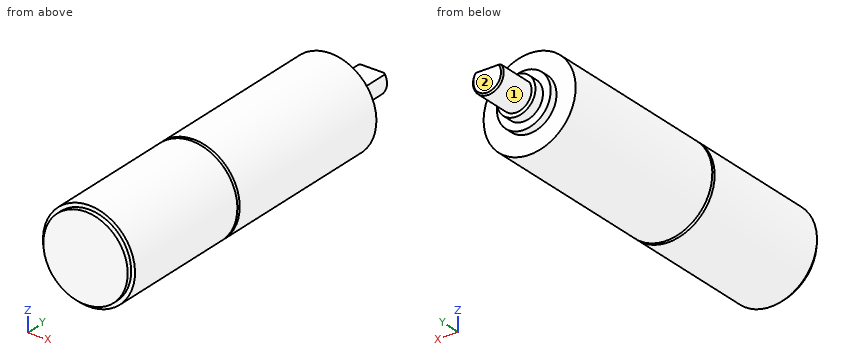
from build123d import *

# Parameters (mm, degrees)
SKETCH_1_R          = 2.75
EXTRUDE_1_DEPTH     = 0.3
EXTRUDE_START       = 0.3
SKETCH_2_R          = 3
EXTRUDE_2_DEPTH     = 9
CHAMFER_1_SIZE      = 0.2
EXTRUDE_START_2     = 9.3
SKETCH_3_R          = 3
EXTRUDE_3_DEPTH     = 11.75
EXTRUDE_START_3     = 21.05
SKETCH_4_R          = 1.75
EXTRUDE_4_DEPTH     = 0.5
SKETCH_5_R          = 1.25
EXTRUDE_5_DEPTH     = 1.15
SKETCH_6_R          = 1
EXTRUDE_6_DEPTH     = 3.65
CUT_EXTRUDE_START   = 22.2
CUT_EXTRUDE_1_DEPTH = 2.5
CHAMFER_2_SIZE      = 0.1


with BuildPart() as part:
    # 草图1 → 凸台-拉伸1 (new body)
    with BuildSketch(Plane(origin=(0, 0, 0), x_dir=(1, 0, 0), z_dir=(0, 1, 0))):
        with Locations(Location((0, 0, 0), (0, 0, 270))):
            Circle(SKETCH_1_R)
    extrude(amount=EXTRUDE_1_DEPTH)

    # 草图2 → 凸台-拉伸2 (add)
    with BuildSketch(Plane(origin=(0, 0, 0), x_dir=(1, 0, 0), z_dir=(0, 1, 0)).offset(EXTRUDE_START)):
        with Locations(Location((0, 0, 0), (0, 0, 270))):
            Circle(SKETCH_2_R)
    extrude(amount=EXTRUDE_2_DEPTH)

    # 倒角1
    chamfer_1_edges = [part.edges().sort_by_distance(p)[0] for p in [
        (0, 9.3, -3),
    ]]
    chamfer(chamfer_1_edges, length=CHAMFER_1_SIZE)

    # 草图3 → 凸台-拉伸3 (add)
    with BuildSketch(Plane(origin=(0, 0, 0), x_dir=(1, 0, 0), z_dir=(0, 1, 0)).offset(EXTRUDE_START_2)):
        with Locations(Location((0, 0, 0), (0, 0, 270))):
            Circle(SKETCH_3_R)
    extrude(amount=EXTRUDE_3_DEPTH)

    # 草图4 → 凸台-拉伸4 (add)
    with BuildSketch(Plane(origin=(0, 0, 0), x_dir=(1, 0, 0), z_dir=(0, 1, 0)).offset(EXTRUDE_START_3)):
        with Locations(Location((0, 0, 0), (0, 0, 270))):
            Circle(SKETCH_4_R)
    extrude(amount=EXTRUDE_4_DEPTH)

    # 草图5 → 凸台-拉伸5 (add)
    with BuildSketch(Plane(origin=(0, 0, 0), x_dir=(1, 0, 0), z_dir=(0, 1, 0)).offset(EXTRUDE_START_3)):
        with Locations(Location((0, 0, 0), (0, 0, 270))):
            Circle(SKETCH_5_R)
    extrude(amount=EXTRUDE_5_DEPTH)

    # 草图6 → 凸台-拉伸6 (add)
    with BuildSketch(Plane(origin=(0, 0, 0), x_dir=(1, 0, 0), z_dir=(0, 1, 0)).offset(EXTRUDE_START_3)):
        with Locations(Location((0, 0, 0), (0, 0, 270))):
            Circle(SKETCH_6_R)
    extrude(amount=EXTRUDE_6_DEPTH)

    # 草图7 → 切除-拉伸1 (cut)
    with BuildSketch(Plane(origin=(0, 0, 0), x_dir=(1, 0, 0), z_dir=(0, 1, 0)).offset(CUT_EXTRUDE_START)):
        with BuildLine():
            Line((-0.866025404, -0.5), (0.866025404, -0.5))
            ThreePointArc((0.866025404, -0.5), (0, -1), (-0.866025404, -0.5))
        make_face()
    extrude(amount=CUT_EXTRUDE_1_DEPTH, mode=Mode.SUBTRACT)

    # 倒角2
    chamfer_2_edges = [part.edges().sort_by_distance(p)[0] for p in [
        (0, 24.7, -1),
    ]]
    chamfer(chamfer_2_edges, length=CHAMFER_2_SIZE)


solid = part.part
CAD build for the part. Positions are in the model's coordinates, mm. Face numbers are marked on the shaded views. A direction names the side the tool comes from. Coordinates: 2 decimals unless noted, no trailing zeros. Order: outer loops, then holes, each group sorted by start corner. A loop starts at its lowest first (then second) coordinate and runs counter-clockwise, first axis right, second up. Notation, with made-up numbers: (-39.5, 38.25) -> (-22.5, 38.25) arc R11 ccw to (-22.5, 42.25) -> close; hole circle Ø2 at (55, 50). An arc over 180 degrees is marked (long way). Answer in a Markdown table with one row per item.
1) Band-saw the part on C-C (y = 7). List the corners of the cut face in (x, z).
Check values:
| item | result |
|---|---|
| outline | circle Ø6 at (0, 0) |
2) Flat gauge pins, fed straight in: P1, Ø2, axis at y = 16, z = 2, coming from the -X side; P2, Ø1.5, axis at y = 11.5, z = 1.5, coming from the +X side; P3, Ø1, axis at x = -1.5, y = 6.5, coming from the -Z side. Where does each tip first touch, or does it go through?
Check values:
| item | result |
|---|---|
| P1 | x = -2.83 |
| P2 | x = 2.9 |
| P3 | z = -2.83 |
3) Band-saw the part on A-A (z = 0). List the corners of the cut face in (x, y), and give its area (3 significant figures).
Check values:
| item | result |
|---|---|
| outline | (-3, 0.3) -> (-2.75, 0.3) -> (-2.75, 0) -> (2.75, 0) -> (2.75, 0.3) -> (3, 0.3) -> (3, 9.1) -> (2.8, 9.3) -> (3, 9.3) -> (3, 21.05) -> (1.75, 21.05) -> (1.75, 21.55) -> (1.25, 21.55) -> (1.25, 22.2) -> (1, 22.2) -> (1, 24.6) -> (0.9, 24.7) -> (-0.9, 24.7) -> (-1, 24.6) -> (-1, 22.2) -> (-1.25, 22.2) -> (-1.25, 21.55) -> (-1.75, 21.55) -> (-1.75, 21.05) -> (-3, 21.05) -> (-3, 9.3) -> (-2.8, 9.3) -> (-3, 9.1) -> close |
| area | 134 mm2 |
4) Which spindle directions (+Z, -Z, +X, -X, +Y, -Y) get a long thin tool onto all of the face, cutting with end or side? Do the marked faces 1 and 2. Say none if no direction does.
Check values:
| item | result |
|---|---|
| face 1 | +Y |
| face 2 | +Z, -Z, +X, -X, +Y |
5) Band-saw the part on B-B (x = 0). List the corners of the cut face in (y, z).
Check values:
| item | result |
|---|---|
| outline | (0, -2.75) -> (0.3, -2.75) -> (0.3, -3) -> (9.1, -3) -> (9.3, -2.8) -> (9.3, -3) -> (21.05, -3) -> (21.05, -1.75) -> (21.55, -1.75) -> (21.55, -1.25) -> (22.2, -1.25) -> (22.2, -1) -> (24.6, -1) -> (24.7, -0.9) -> (24.7, 0.5) -> (22.2, 0.5) -> (22.2, 1.25) -> (21.55, 1.25) -> (21.55, 1.75) -> (21.05, 1.75) -> (21.05, 3) -> (9.3, 3) -> (9.3, 2.8) -> (9.1, 3) -> (0.3, 3) -> (0.3, 2.75) -> (0, 2.75) -> close |
6) Drill centre lines: line 1 (Y direction, x = 1.6, z = -2.2); line 2 (Y direction, x = 0.6, z = 0.9); line 3 (X direction, y = 16.75, z = -0.2). Where is each one in solid material? Low to high.
Check values:
| item | result |
|---|---|
| line 1 | 0 to 21.05 |
| line 2 | 0 to 22.2 |
| line 3 | -2.99 to 2.99 |
